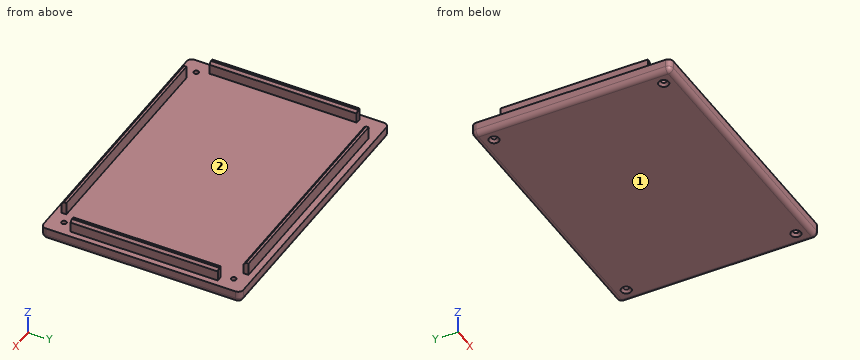
```python
from build123d import *

# Parameters (mm, degrees)
SKETCH_W        = 110
SKETCH_H        = 80
PAD_DEPTH       = 5
SKETCH001_R     = 1
POCKET_DEPTH    = 5
CHAMFER_SIZE    = 1
SKETCH002_W     = 89
SKETCH002_H     = 2
SKETCH002_W_2   = 2
SKETCH002_H_2   = 59
PAD001_DEPTH    = 5
CHAMFER001_SIZE = 1
FILLET_R        = 2


with BuildPart() as part:
    # Sketch → Pad (new body)
    with BuildSketch(Plane.XY):
        Rectangle(SKETCH_W, SKETCH_H)
    extrude(amount=PAD_DEPTH)

    # Sketch001 (on Face6 of Pad) → Pocket (cut)
    with BuildSketch(Plane.XY.offset(5)):
        with Locations((49, 34)):
            Circle(SKETCH001_R)
        with Locations((-49, 34)):
            Circle(SKETCH001_R)
        with Locations((-49, -34)):
            Circle(SKETCH001_R)
        with Locations((49, -34)):
            Circle(SKETCH001_R)
    extrude(amount=-POCKET_DEPTH, mode=Mode.SUBTRACT)

    # Chamfer
    chamfer_edges = [part.edges().sort_by_distance(p)[0] for p in [
        (-50, -34, 0),
        (-50, 34, 0),
        (48, 34, 0),
        (48, -34, 0),
    ]]
    chamfer(chamfer_edges, length=CHAMFER_SIZE)

    # Sketch002 (on Face11 of Chamfer) → Pad001 (join)
    with BuildSketch(Plane.XY.offset(5)):
        with Locations((0, 36.5)):
            Rectangle(SKETCH002_W, SKETCH002_H)
        with Locations((0, -36.5)):
            Rectangle(SKETCH002_W, SKETCH002_H)
        with Locations((51.5, 0)):
            Rectangle(SKETCH002_W_2, SKETCH002_H_2)
        with Locations((-51.5, 0)):
            Rectangle(SKETCH002_W_2, SKETCH002_H_2)
    extrude(amount=PAD001_DEPTH)

    # Chamfer001
    chamfer001_edges = [part.edges().sort_by_distance(p)[0] for p in [
        (0, 35.5, 10),
        (52.5, 0, 10),
        (-50.5, 0, 10),
        (0, -37.5, 10),
    ]]
    chamfer(chamfer001_edges, length=CHAMFER001_SIZE)

    # Fillet
    fillet_edges = [part.edges().sort_by_distance(p)[0] for p in [
        (-55, -40, 2.5),
        (-55, 0, 0),
        (-55, 40, 2.5),
        (0, 40, 0),
        (55, 40, 2.5),
        (55, 0, 0),
        (55, -40, 2.5),
        (0, -40, 0),
    ]]
    fillet(fillet_edges, radius=FILLET_R)


solid = part.part
```
Work out the finished part from the listing and answer in its coordinate system (mm). Face numbers are marked on the shaded views. Coordinates: 2 decimals unless noted, no trailing zeros. Loops run counter-clockwise (first coordinate to the right, second up) from the corner with the lowest first, then second, coordinate; pieces in that order, holes last. Notation, with made-up numbers: M 26.25,50 L 59.25,50 A25 ccw 59.25,65 Z; hole C 81,46 d7. An arc over 180 degrees is marked long. Use CSV: the item, a comma, the result in double quotes. Start each with the question number.
(1) Given pin 1 Ø0.6 at (x, z) = (-51, 7) entering from +Y; pin 2 Ø1.6 at (y, z) = (36.5, 8) entering from -X; pin 3 Ø3 at (y, z) = (-30.5, 8.5) entering from -X, each flat-ended and moving along its own axis, determine where each tip first touches the part or whether it passes through.
(2) Find section B-B, the plane x = 17.5. Give the vertices of the cut face in (y, z).
(3) For a pull along X with two mould halves and no side action, classify the marked faces 1 and 2 as +X half, -X half, draft (parallel to the pull), parting line (faces both ways), or undercut.
(4) Find section A-A, the plane y = 6.5. Give the vertices of the cut face in (x, z).
(5) Consider line 1 (Y direction, x = -8.5, z = 6.5); line 2 (X direction, y = 13, z = 8.5); line 3 (Z direction, x = -9.5, y = -15). Determine where each line is inside the solid, lowest interval first.
Recorded:
1,pin 1,"stops at y = 29.5"
1,pin 2,"stops at x = -44.5"
1,pin 3,"stops at x = -52.5"
2,outline,"M -40,2 A2 ccw -38,0 L 38,0 A2 ccw 40,2 L 40,5 L 37.5,5 L 37.5,10 L 36.5,10 L 35.5,9 L 35.5,5 L -35.5,5 L -35.5,10 L -36.5,10 L -37.5,9 L -37.5,5 L -40,5 Z"
3,face 1,"draft"
3,face 2,"undercut"
4,outline,"M -55,2 A2 ccw -53,0 L 53,0 A2 ccw 55,2 L 55,5 L 52.5,5 L 52.5,9 L 51.5,10 L 50.5,10 L 50.5,5 L -50.5,5 L -50.5,9 L -51.5,10 L -52.5,10 L -52.5,5 L -55,5 Z"
5,line 1,"y = -37.5 to -35.5, 35.5 to 37.5"
5,line 2,"x = -52.5 to -50.5, 50.5 to 52.5"
5,line 3,"z = 0 to 5"
